Design review of the part built by this model. Coordinates are the model's own, in mm. Give positions to 0.01 mm unless a question says otherwise; leave off trailing zeros. Loops run counter-clockwise (first coordinate to the right, second up) from the corner with the lowest first, then second, coordinate; pieces in that order, holes last. Notation, with made-up numbers: (11.25, 21) -> (55.25, 21) arc R12 cw to (55.25, 33) -> close; hole circle Ø8 at (51, 86). An arc over 180 degrees is marked (long way). Answer in a Markdown table with one row per item. Add a question column.
(1) Draft analysis for pull direction X (two halves, no side actions). For faces 1 (the cylindrical face through (13.28, 260.3, 1.57)), 2 (the flat face through (23.77, 289.24, 1.57)), 3 (the flat face through (32, 232, 3.175)), state which applies: +X half, -X half, draft (parallel to the pull), parting line (faces both ways), or undercut.
(2) Consider section B-B on y = 206. Write out the cut boundary in (x, z) (3 decimals).
(3) Consider section A-A on z = 0.7. Write out the cut boundary in (x, y) (3 decimals).
(4) Consider section C-C on y = 228. Write out the cut boundary in (x, z) (3 decimals).
(5) For pin 1 (1.5 mm diameter, centred on x = 67.5, z = 2.5, fed in from -Y); pin 2 (6.5 mm diameter, centred on x = 32.74, y = 283.14, fed in from +Z) (3 decimals); pin 3 (1.5 mm diameter, centred on x = 48, z = 1, fed in from -Y); pin 4 (3 mm diameter, centred on x = 12.7, y = 238.125, fed in from +Z), all flat-tipped, find the tip position at first contact; note any pin that passes through.
(6) For line 1 (Y direction, x = 16.5, z = 0.7); line 2 (Y direction, x = 14.5, z = 0.9); line 3 (Y direction, x = 31, z = 2.05), list the stretches that pass through material, from the lowest coordinate up.
from build123d import *

# Parameters (mm, degrees)
BOSS_EXTRUDE1_DEPTH    = 3.175
F_10_CLEARANCE_HOLE1_D = 4.9784


with BuildPart() as part:
    # Sketch2 → Boss-Extrude1 (new body)
    with BuildSketch(Plane.XY):
        Polygon((75.96605069, 191.201454104), (42.169306363, 295.217137729), (4.854209552, 283.092727808), (4.854209552, 203.901454104), align=None)
    extrude(amount=BOSS_EXTRUDE1_DEPTH)

    # #10 Clearance Hole1 (through all)
    with Locations(Plane.XY.offset(3.175)):
        with Locations((32.740251946, 283.138719963), (59.435154755, 200.980257064), (12.7, 238.125), (12.7, 212.725), (14.622625311, 277.25194622), (14.622625311, 258.20194622)):
            Hole(F_10_CLEARANCE_HOLE1_D / 2)


solid = part.part
Values follow:
| question | item | result |
|---|---|---|
| 1 | face 1 | undercut |
| 1 | face 2 | -X half |
| 1 | face 3 | draft |
| 2 | outline | (4.854, 0) -> (71.158, 0) -> (71.158, 3.175) -> (4.854, 3.175) -> close |
| 3 | outline | (4.854, 203.901) -> (75.966, 191.201) -> (42.169, 295.217) -> (4.854, 283.093) -> close; hole circle Ø4.978 at (12.7, 212.725); hole circle Ø4.978 at (12.7, 238.125); hole circle Ø4.978 at (14.623, 258.202); hole circle Ø4.978 at (14.623, 277.252); hole circle Ø4.978 at (32.74, 283.139); hole circle Ø4.978 at (59.435, 200.98) |
| 4 | outline | (4.854, 0) -> (64.009, 0) -> (64.009, 3.175) -> (4.854, 3.175) -> close |
| 5 | pin 1 | y = 192.58 |
| 5 | pin 2 | z = 3.175 |
| 5 | pin 3 | y = 196.06 |
| 5 | pin 4 | through |
| 6 | line 1 | 201.82 to 256.57, 259.84 to 275.62, 278.89 to 286.88 |
| 6 | line 2 | 202.18 to 211.01, 214.44 to 236.41, 239.84 to 255.72, 260.69 to 274.77, 279.74 to 286.23 |
| 6 | line 3 | 199.23 to 281.36, 284.92 to 291.59 |
